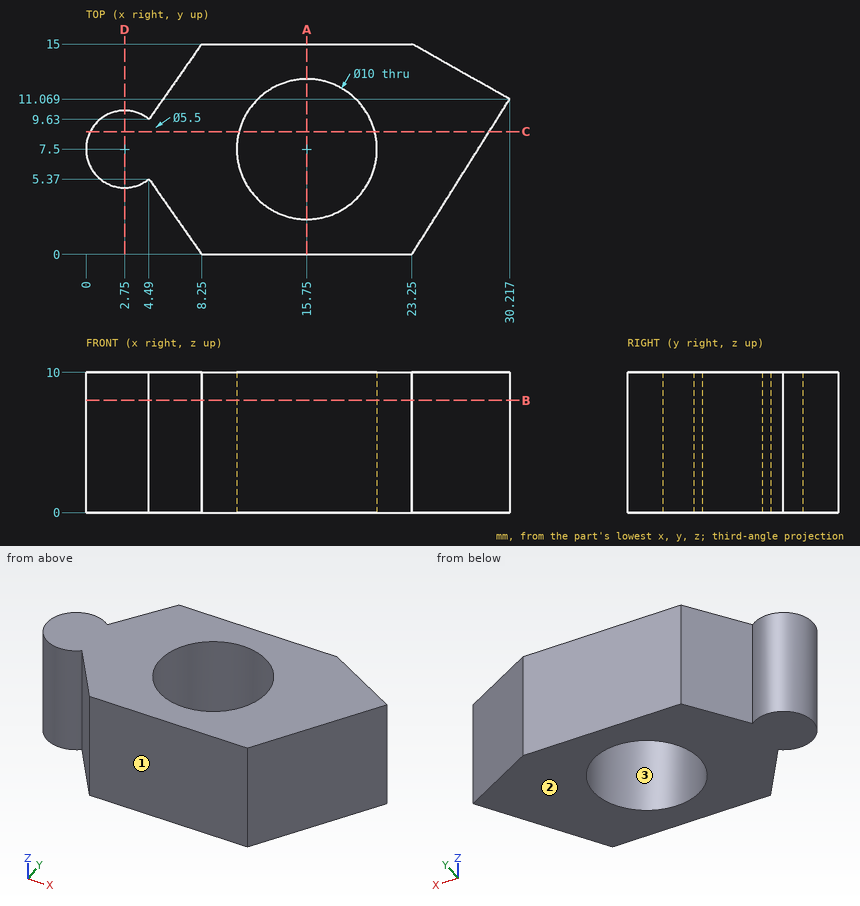
For this review, use the dimensioned drawing (mm, ordinates from the lowest corner) and the shaded views. Give positions to 0.01 mm unless a question says otherwise; leave off trailing zeros. Order: outer loops, then holes, each group sorted by start corner. A loop starts at its lowest first (then second) coordinate and runs counter-clockwise, first axis right, second up. Notation, with made-up numbers: M 58.25,74.25 L 95.25,74.25 A22 ccw 95.25,82.25 Z; hole C 60.5,7.25 d6. An arc over 180 degrees is marked long. One line per question, with ' | ' between items. Start each with the question number.
1) Consider section A-A, the plane x = 15.75. Give the boundary of the cut face in (y, z).
2) Consider section C-C, the plane y = 8.75. Give the boundary of the cut face in (x, z).
3) Clearance check with flat-ended pins moving along their axes: P1, Ø1, axis at x = 15.5, y = 10, coming from the -Z side; P2, Ø4, axis at y = 4, z = 8.5, coming from the +X side; P3, Ø4, axis at y = 6, z = 5, coming from the +X side (1 decimal); P4, Ø1, axis at y = 9, z = 3.5, coming from the +X side. State where each tip first meets the part, or that it passes through.
4) Consider section B-B, the plane z = 8. Give the boundary of the cut face in (x, y).
5) Consider section D-D, the plane x = 2.75. Give the boundary of the cut face in (y, z).
6) Mouldability with a two-part tool opening along Y and no side actions: class the marked faces 1, 2 and 3 as pulls with the +Y half, pulls with the -Y half, needs draft (parallel to the pull), parting line crosses it, or undercut.
7) Wall thickness on L1, parallel to Y at x = 15.75, z = 5.5; L2, parallel to X at y = 10.5, z = 9.75; L3, parallel to X at y = 8.75, z = 6.5: over which ranges is each line inside the solid? List them lowest first. Write a range as from..to.
Found:
1) outline: M 0,0 L 2.5,0 L 2.5,10 L 0,10 Z; M 12.5,0 L 15,0 L 15,10 L 12.5,10 Z
2) outline: M 0.3,0 L 10.91,0 L 10.91,10 L 0.3,10 Z; M 20.59,0 L 28.76,0 L 28.76,10 L 20.59,10 Z
3) P1: passes through | P2: stops at x = 27.03 | P3: stops at x = 28.3 | P4: stops at x = 29.23
4) outline: M 4.49,5.37 L 8.25,0 L 23.25,0 L 30.22,11.07 L 23.25,15 L 8.25,15 L 4.49,9.63 A2.75 ccw long Z; hole C 15.75,7.5 d10
5) outline: M 4.75,0 L 10.25,0 L 10.25,10 L 4.75,10 Z
6) face 1: pulls with the -Y half | face 2: needs draft | face 3: undercut
7) L1: y = 0..2.5, 12.5..15 | L2: x = 5.1..11.75, 19.75..29.86 | L3: x = 0.3..10.91, 20.59..28.76
